The drawing under review shows one solid part. Ordinate dimensions are in mm from its lowest x, y, z. A direction names the side the tool comes from. Coordinates: 2 decimals unless noted, no trailing zeros. Loops run counter-clockwise (first coordinate to the right, second up) from the corner with the lowest first, then second, coordinate; pieces in that order, holes last. Notation, with made-up numbers: (70.5, -4) - (118.5, -4) arc R14 ccw to (118.5, 20) - close; hole circle Ø4 at (-22.5, -31.75). An arc over 180 degrees is marked (long way). Use one line per item in the form item = value. Start each with the question number.
1. To check wall thickness, follow probe 1 along X at (y, z) = (229.5, 227.5); probe 2 along Y at (x, z) = (974.5, 52); probe 3 along Z at (x, y) = (508, 188.5). State the ranges of each line that lie inside material, in increasing order.
2. Add section D-D on z = 54.5. Give the boundary of the cut face in (x, y).
3. Machinability: for the marked faces 1, 2 and 3, which of the approach directions +Z, -Z, +X, -X, +Y, -Y give a long, thin tool a straight path to every point of the face, cutting with its end or side? Answer none if there is none.
4. Add section A-A on z = 152.4. Give the boundary of the cut face in (x, y), and give its area (3 significant figures).
5. Add section C-C on x = 470.5. Give the boundary of the cut face in (y, z).
6. For pin 1 Ø6 at (x, y) = (812, 137.5) entering from -Z; pin 2 Ø1.5 at (x, y) = (425, 56.5) entering from +Z; pin 3 Ø6 at (x, z) = (775, 247.5) entering from -Y, all flat-tipped, find the tip position at first contact; note any pin that passes through.
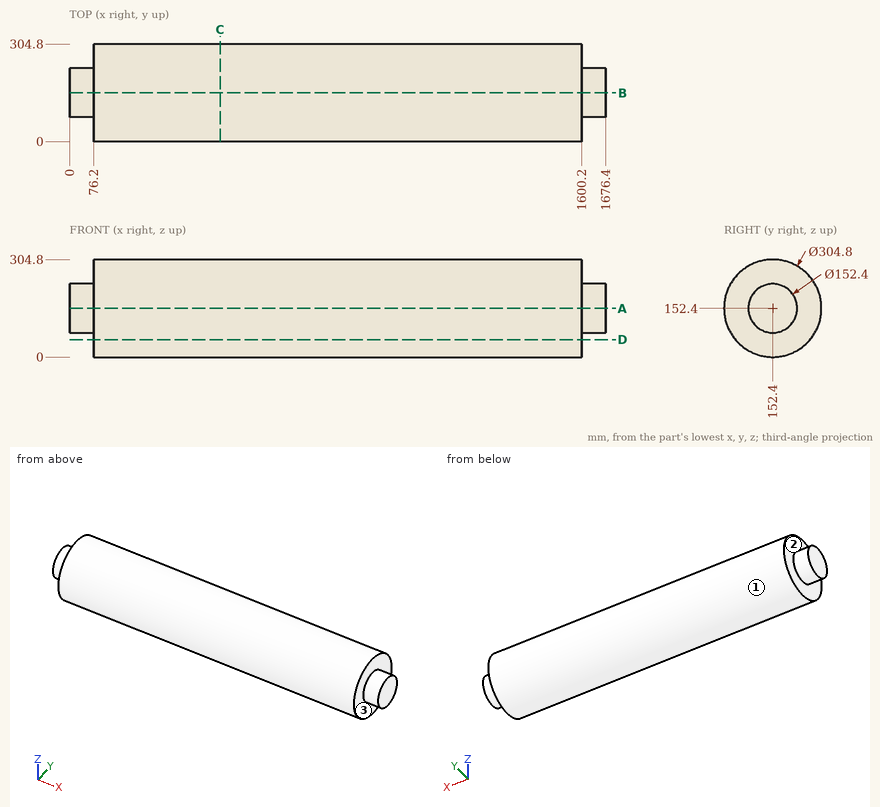
Conclusion:
q1.probe_1 = 76.2 to 1600.2
q1.probe_2 = 37.75 to 267.05
q1.probe_3 = 4.34 to 300.46
q2.outline = (76.2, 35.6) - (1600.2, 35.6) - (1600.2, 269.2) - (76.2, 269.2) - close
q3.face_1 = +X, -X
q3.face_2 = -X
q3.face_3 = +X
q4.outline = (0, 76.2) - (76.2, 76.2) - (76.2, 0) - (1600.2, 0) - (1600.2, 76.2) - (1676.4, 76.2) - (1676.4, 228.6) - (1600.2, 228.6) - (1600.2, 304.8) - (76.2, 304.8) - (76.2, 228.6) - (0, 228.6) - close
q4.area = 488,000 mm^2
q5.outline = circle Ø304.8 at (152.4, 152.4)
q6.pin_1 = 0.47
q6.pin_2 = 271.45
q6.pin_3 = 30.98
